from build123d import *

# Parameters (mm, degrees)
BOSS_EXTRUDE1_DEPTH = 6
SKETCH2_W           = 116
SKETCH2_H           = 265
BOSS_EXTRUDE2_DEPTH = 6
SKETCH3_R           = 10
CUT_EXTRUDE1_DEPTH  = 6


with BuildPart() as part:
    # Sketch1 → Boss-Extrude1 (new body)
    with BuildSketch(Plane.XY):
        Polygon((68, 245), (48, 245), (48, 0), (-48, 0), (-48, -20), (68, -20), align=None)
    extrude(amount=-BOSS_EXTRUDE1_DEPTH)

    # Sketch2 → Boss-Extrude2 (add)
    with BuildSketch(Plane.XY):
        with Locations((10, 112.5)):
            Rectangle(SKETCH2_W, SKETCH2_H)
    extrude(amount=BOSS_EXTRUDE2_DEPTH)

    # Sketch3 → Cut-Extrude1 (cut)
    with BuildSketch(Plane(origin=(0, 0, -6), x_dir=(-1, 0, 0), z_dir=(0, 0, -1))):
        with Locations((-48, 0)):
            Circle(SKETCH3_R)
    extrude(amount=-CUT_EXTRUDE1_DEPTH, mode=Mode.SUBTRACT)


solid = part.part
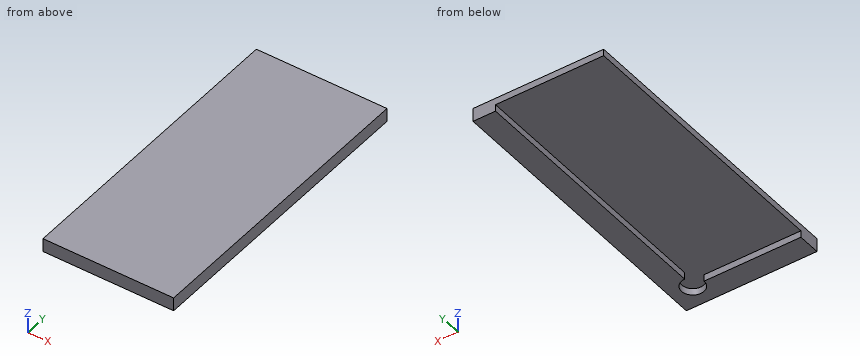
Read the model definition and answer for the solid it produces. Units are mm, in the model's axes. Give positions to 0.01 mm unless a question says otherwise; leave off trailing zeros. Write each loop counter-clockwise with the first axis right and the second up, starting at its lowest first coordinate (ties: lowest second). Pieces come first, ordered by that corner, then holes. Notation, with made-up numbers: (35.25, 31.25) - (58.25, 31.25) arc R26 ccw to (58.25, 69.25) - close; hole circle Ø3 at (36.5, 44.5). An arc over 180 degrees is marked (long way). Use CSV: the item, a comma, the result in double quotes. Start each with the question number.
Item 1: The part is cut by section B-B, the plane x = 9.5. Give the vertices of the cut face in (y, z), and give its area (3 significant figures).
Item 2: The part is cut by section A-A, the plane y = 75. Give the vertices of the cut face in (x, z), and give its area (3 significant figures).
Item 3: Consider line 1 (Y direction, x = -27, z = -3.75); line 2 (Z direction, x = -29.5, y = 28.5); line 3 (X direction, y = 109, z = -3). Determine where each line is inside the solid, lowest interval first.
Item 4: Flat-ended cylindrical pins translate along their axes: P1, Ø16, axis at x = 48, y = 0, coming from the -Z side; P2, Ø3, axis at y = 113, z = -2, coming from the -X side; P3, Ø1.5, axis at x = 45, z = -4, coming from the +Y side. Find the tip coordinate at first contact, or state that the pin passes through.
Item 5: The part is cut by section C-C, the plane z = -2.5. Give the vertices of the cut face in (x, y), and give its area (3 significant figures).
Taken from the geometry:
1,outline,"(-20, -6) - (0, -6) - (0, 0) - (245, 0) - (245, 6) - (-20, 6) - close"
1,area,"1,710 mm2"
2,outline,"(-48, 0) - (48, 0) - (48, -6) - (68, -6) - (68, 6) - (-48, 6) - close"
2,area,"816 mm2"
3,line 1,"-20 to 0"
3,line 2,"0 to 6"
3,line 3,"48 to 68"
4,P1,"z = 0"
4,P2,"x = 48"
4,P3,"y = -9.27"
5,outline,"(-48, -20) - (68, -20) - (68, 245) - (48, 245) - (48, 10) arc R10 cw (long way) to (38, 0) - (-48, 0) - close"
5,area,"6,980 mm2"
